```python
from build123d import *

# Parameters (mm, degrees)
SKETCH1_W            = 200
SKETCH1_H            = 30
BASE_DEPTH           = 6.35
WEDGECUT_REACH       = 202.662
SKETCH3_W            = 40
SKETCH3_H            = 8
HINGE_CUTOUT_DEPTH   = 0.635
HINGE_HOLE_CUT_REACH = 103.28
SKETCH4_R            = 1.8034
SKETCH5_W            = 5.05
SKETCH5_H            = 5.05
HINGE_NUT_CUT_DEPTH  = 2
SKETCH6_R            = 5.08
CUT_EXTRUDE1_DEPTH   = 102.317927831
SKETCH7_R            = 5.08
SKETCH7_R_2          = 2.54
BOSS_EXTRUDE1_DEPTH  = 1


with BuildPart() as part:
    # Sketch1 → Base (new body)
    with BuildSketch(Plane(origin=(0, 0, 0), x_dir=(1, 0, 0), z_dir=(0, 1, 0))):
        Rectangle(SKETCH1_W, SKETCH1_H)
    extrude(amount=BASE_DEPTH)

    # Sketch2 → WedgeCut (cut, up to next)
    with BuildSketch(Plane(origin=(100, 0, 0), x_dir=(0, 0, -1), z_dir=(1, 0, 0)), mode=Mode.PRIVATE) as wedgecut_sk1:
        Polygon((-15, 0), (-6.907470508, 0), (8.342084542, 5.407501552), (8.007874016, 6.35), (-15, 6.35), align=None)
    wedgecut_tool1 = extrude(wedgecut_sk1.sketch, amount=-WEDGECUT_REACH, mode=Mode.PRIVATE) & part.part
    add(wedgecut_tool1.solids().sort_by_distance((100, 3.70048, 5.888491))[0], mode=Mode.SUBTRACT)

    # Sketch3 → Hinge Cutout (cut)
    with BuildSketch(Plane(origin=(0, 6.35, 0), x_dir=(1, 0, 0), z_dir=(0, 1, 0))):
        with Locations((-69.999999934, 11)):
            Rectangle(SKETCH3_W, SKETCH3_H)
        with Locations((70, 11)):
            Rectangle(SKETCH3_W, SKETCH3_H)
    extrude(amount=-HINGE_CUTOUT_DEPTH, mode=Mode.SUBTRACT)

    # Sketch4 → Hinge Hole Cut (cut, up to next)
    with BuildSketch(Plane(origin=(0, 5.715, 0), x_dir=(1, 0, 0), z_dir=(0, 1, 0)), mode=Mode.PRIVATE) as hinge_hole_cut_sk1:
        with Locations(Location((54, 11.825, 0), (0, 0, 270))):
            Circle(SKETCH4_R)
    hinge_hole_cut_tool1 = extrude(hinge_hole_cut_sk1.sketch, amount=-HINGE_HOLE_CUT_REACH, mode=Mode.PRIVATE) & part.part
    # Sketch4 → Hinge Hole Cut (cut, up to next)
    with BuildSketch(Plane(origin=(0, 5.715, 0), x_dir=(1, 0, 0), z_dir=(0, 1, 0)), mode=Mode.PRIVATE) as hinge_hole_cut_sk2:
        with Locations(Location((84, 11.825, 0), (0, 0, 270))):
            Circle(SKETCH4_R)
    hinge_hole_cut_tool2 = extrude(hinge_hole_cut_sk2.sketch, amount=-HINGE_HOLE_CUT_REACH, mode=Mode.PRIVATE) & part.part
    hinge_hole_cut_1 = hinge_hole_cut_tool1.solids().sort_by_distance((54, 5.715, -11.825))[0]
    add(hinge_hole_cut_1, mode=Mode.SUBTRACT)
    hinge_hole_cut_2 = hinge_hole_cut_tool2.solids().sort_by_distance((84, 5.715, -11.825))[0]
    add(hinge_hole_cut_2, mode=Mode.SUBTRACT)
    hinge_hole_cut = hinge_hole_cut_1 + hinge_hole_cut_2  # Hinge Hole Cut as one shape, for the pattern or mirror that repeats it

    # Sketch5 → Hinge Nut Cut (cut)
    with BuildSketch(Plane.XZ):
        with Locations((54, -11.825)):
            Rectangle(SKETCH5_W, SKETCH5_H)
        with Locations((84, -11.825)):
            Rectangle(SKETCH5_W, SKETCH5_H)
    hinge_nut_cut = extrude(amount=-HINGE_NUT_CUT_DEPTH, mode=Mode.SUBTRACT)

    # Hinge Hole Mirror: Hinge Hole Cut, Hinge Nut Cut across plane
    add(hinge_hole_cut.mirror(Plane(origin=(0, 0, 0), x_dir=(0, 0, 1), z_dir=(1, 0, 0))), mode=Mode.SUBTRACT)
    add(hinge_nut_cut.mirror(Plane(origin=(0, 0, 0), x_dir=(0, 0, 1), z_dir=(1, 0, 0))), mode=Mode.SUBTRACT)

    # Sketch6 → Cut-Extrude1 (cut, through all)
    with BuildSketch(Plane(origin=(0, 0, 0), x_dir=(-1, 0, 0), z_dir=(0, -1, 0))):
        with Locations(Location((-80, 5, 0), (0, 0, 106.879170472))):
            Circle(SKETCH6_R)
        with Locations(Location((-40, 5, 0), (0, 0, 90))):
            Circle(SKETCH6_R)
        with Locations(Location((0, 5, 0), (0, 0, 90))):
            Circle(SKETCH6_R)
        with Locations(Location((40, 5, 0), (0, 0, 90))):
            Circle(SKETCH6_R)
        with Locations(Location((80, 5, 0), (0, 0, 73.120829528))):
            Circle(SKETCH6_R)
    extrude(amount=-CUT_EXTRUDE1_DEPTH, mode=Mode.SUBTRACT)

    # Sketch7 → Boss-Extrude1 (add)
    # profile 1 of 5: a face of its own
    with BuildSketch(Plane.XZ):
        with Locations(Location((-80, -5, 0), (0, 0, 253.120829528))):
            Circle(SKETCH7_R)
        with Locations(Location((-80, -5, 0), (0, 0, 270))):
            Circle(SKETCH7_R_2, mode=Mode.SUBTRACT)
    # profile 2 of 5: a face of its own
    with BuildSketch(Plane.XZ):
        with Locations(Location((-40, -5, 0), (0, 0, 270))):
            Circle(SKETCH7_R)
        with Locations(Location((-40, -5, 0), (0, 0, 270))):
            Circle(SKETCH7_R_2, mode=Mode.SUBTRACT)
    # profile 3 of 5: a face of its own
    with BuildSketch(Plane.XZ):
        with Locations(Location((0, -5, 0), (0, 0, 270))):
            Circle(SKETCH7_R)
        with Locations(Location((0, -5, 0), (0, 0, 270))):
            Circle(SKETCH7_R_2, mode=Mode.SUBTRACT)
    # profile 4 of 5: a face of its own
    with BuildSketch(Plane.XZ):
        with Locations(Location((40, -5, 0), (0, 0, 270))):
            Circle(SKETCH7_R)
        with Locations(Location((40, -5, 0), (0, 0, 270))):
            Circle(SKETCH7_R_2, mode=Mode.SUBTRACT)
    # profile 5 of 5: a face of its own
    with BuildSketch(Plane.XZ):
        with Locations(Location((80, -5, 0), (0, 0, 286.879170472))):
            Circle(SKETCH7_R)
        with Locations(Location((80, -5, 0), (0, 0, 270))):
            Circle(SKETCH7_R_2, mode=Mode.SUBTRACT)
    extrude(amount=-BOSS_EXTRUDE1_DEPTH)


solid = part.part
```
The listing builds one solid part. Answer for the finished solid, in the listing's coordinates (mm). A direction names the side the tool comes from. Coordinates: 2 decimals unless noted, no trailing zeros. Write each loop counter-clockwise with the first axis right and the second up, starting at its lowest first coordinate (ties: lowest second). Pieces come first, ordered by that corner, then holes. Notation, with made-up numbers: (20.25, -36.5) - (47.25, -36.5) arc R30 cw to (47.25, -14.5) - close; hole circle Ø6 at (21, 54.25). An arc over 180 degrees is marked (long way). Return JSON: item names as keys, results as strings. Group by question number.
Q1. The part is cut by section C-C on z = -5. State how many separate pieces and enclosed holes the cut face has, and give its area (3 significant figures).
Q2. Flat-ended cylindrical pins translate along their axes: pin 1 Ø8 at (x, z) = (-40, -5) entering from +Y; pin 2 Ø5 at (x, z) = (46, 4) entering from +Y; pin 3 Ø11 at (x, z) = (-78.5, -7) entering from +Y (3 decimals); pin 4 Ø1.5 at (x, z) = (-53, -12) entering from -Y. Find the tip coordinate at first contact, or state that the pin passes through.
Q3. The part is cut by section D-D on x = 0. Write down the section's boundary in (y, z), and give its area (3 significant figures).
Q4. Which of the six approach directions +Z, -Z, +X, -X, +Y, -Y give full straight-line access (tool end or side, diameter ignored) to faces 1 (the flat face through (70, 5.715, -12)), 2 (the flat face through (83, 2, -10)), 3 (the cylindrical face through (-41.95, 3.04, -9.69))?
Q5. For a pull along X with two mould halves and no side action, classify faces 4 (the flat face through (-95, 6.35, -12)), 5 (the flat face through (-100, 2, -6)), 6 (the cylindrical face through (82.52, 0.49, -4.67)) as +X half, -X half, draft (parallel to the pull), parting line (faces both ways), or undercut.
Q6. Find the intervals of material crossed by line 1 along X through (y, z) = (0.65, -5); line 2 along X through (y, z) = (0.75, -13.75) (3 decimals); line 3 along X through (y, z) = (2.3, -5), in increasing order. Write a range as [from, to].
Evaluation:
{
 "1": {"separate pieces": "6", "enclosed holes": "0", "area": "655 mm2"},
 "2": {"pin 1": "stops at y = 1", "pin 2": "stops at y = 1.92", "pin 3": "stops at y = 5.715", "pin 4": "passes through"},
 "3": {"outline": "(0, -15) - (6.35, -15) - (6.35, -10.08) - (1, -10.08) - (1, -7.54) - (0, -7.54) - close; (0, -2.46) - (1, -2.46) - (1, 0.08) - (2.42, 0.08) - (0, 6.91) - close", "area": "44.6 mm2"},
 "4": {"face 1": "+Z, -Z, +Y", "face 2": "-Y", "face 3": "+Y"},
 "5": {"face 4": "draft", "face 5": "-X half", "face 6": "undercut"},
 "6": {"line 1": "x = [-100, -82.54], [-77.46, -42.54], [-37.46, -2.54], [2.54, 37.46], [42.54, 77.46], [82.54, 100]", "line 2": "x = [-100, -86.525], [-81.475, -56.525], [-51.475, 51.475], [56.525, 81.475], [86.525, 100]", "line 3": "x = [-100, -85.08], [-74.92, -45.08], [-34.92, -5.08], [5.08, 34.92], [45.08, 74.92], [85.08, 100]"}
}
